For this review, take the finished solid that the model builds, in its own axes (mm). Face numbers are marked on the shaded views. A direction names the side the tool comes from. Coordinates: 2 decimals unless noted, no trailing zeros. Order: outer loops, then holes, each group sorted by start corner. A loop starts at its lowest first (then second) coordinate and runs counter-clockwise, first axis right, second up. Notation, with made-up numbers: (14, 2) -> (46, 2) arc R30 cw to (46, 36) -> close; hole circle Ø2 at (51, 79). An arc over 180 degrees is marked (long way). Answer as a JSON object with one key per item and string values. Group by question number.
1) Add section B-B, the plane z = 61. Write out the cut boundary in (x, y).
2) For pin 1 (5.5 mm diameter, centred on x = 36.5, y = 13.5, fed in from +Z); pin 2 (12 mm diameter, centred on y = -9, z = 47.5, fed in from -X); pin 3 (8 mm diameter, centred on y = -12.5, z = 17, fed in from -X); pin 4 (4 mm diameter, centred on x = 54, z = 52.5, fed in from -Y), all flat-tipped, find the tip position at first contact; note any pin that passes through.
3) Draft analysis for pull direction X (two halves, no side actions). For the marked faces 4, 5, 6 and 7, state which applies: +X half, -X half, draft (parallel to the pull), parting line (faces both ways), or undercut.
4) Wall thickness on L1, parallel to Y at x = 35, z = 22; L2, parallel to Y at x = 9, z = 38; L3, parallel to X at y = 9, z = 58: over which ranges is each line inside the solid? List them lowest first.
5) Add section D-D, the plane x = 32.5. Write out the cut boundary in (y, z).
6) Add section C-C, the plane y = -20.5. Write out the cut boundary in (x, z).
7) Machinability: for the marked faces 1, 2 and 3, which of the approach directions +Z, -Z, +X, -X, +Y, -Y give a long, thin tool a straight path to every point of the face, cutting with its end or side? Answer none if there is none.
8) Add section A-A, the plane z = 29. Write out the cut boundary in (x, y), then the cut area to 3 significant figures.
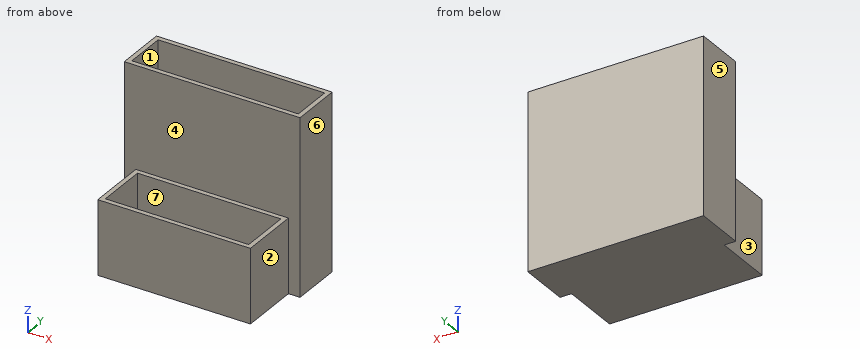
from build123d import *

# Parameters (mm, degrees)
SKETCH_W        = 76
SKETCH_H        = 22
PAD_DEPTH       = 76
SKETCH001_W     = 66
SKETCH001_H     = 26
PAD001_DEPTH    = 32
SKETCH002_W     = 62
SKETCH002_H     = 22
POCKET_DEPTH    = 30
SKETCH003_W     = 72
SKETCH003_H     = 18
POCKET001_DEPTH = 74


with BuildPart() as part:
    # Sketch → Pad (new body)
    with BuildSketch(Plane.XY):
        with Locations((38, 11)):
            Rectangle(SKETCH_W, SKETCH_H)
    extrude(amount=PAD_DEPTH)

    # Sketch001 → Pad001 (join)
    with BuildSketch(Plane.XY):
        with Locations((38, -13)):
            Rectangle(SKETCH001_W, SKETCH001_H)
    extrude(amount=PAD001_DEPTH)

    # Sketch002 (on Face4 of Pad001) → Pocket (cut)
    with BuildSketch(Plane.XY.offset(32)):
        with Locations((38, -13)):
            Rectangle(SKETCH002_W, SKETCH002_H)
    extrude(amount=-POCKET_DEPTH, mode=Mode.SUBTRACT)

    # Sketch003 (on Face7 of Pocket) → Pocket001 (cut)
    with BuildSketch(Plane.XY.offset(76)):
        with Locations((38, 11)):
            Rectangle(SKETCH003_W, SKETCH003_H)
    extrude(amount=-POCKET001_DEPTH, mode=Mode.SUBTRACT)


solid = part.part
Output values:
{
 "1": {"outline": "(0, 0) -> (76, 0) -> (76, 22) -> (0, 22) -> close; hole (2, 2) -> (74, 2) -> (74, 20) -> (2, 20) -> close"},
 "2": {"pin 1": "stops at z = 2", "pin 2": "passes through", "pin 3": "stops at x = 5", "pin 4": "stops at y = 0"},
 "3": {"face 4": "draft", "face 5": "-X half", "face 6": "+X half", "face 7": "undercut"},
 "4": {"L1": "y = -26 to -24, -2 to 2, 20 to 22", "L2": "y = 0 to 2, 20 to 22", "L3": "x = 0 to 2, 74 to 76"},
 "5": {"outline": "(-26, 0) -> (22, 0) -> (22, 76) -> (20, 76) -> (20, 2) -> (2, 2) -> (2, 76) -> (0, 76) -> (0, 32) -> (-2, 32) -> (-2, 2) -> (-24, 2) -> (-24, 32) -> (-26, 32) -> close"},
 "6": {"outline": "(5, 0) -> (71, 0) -> (71, 32) -> (69, 32) -> (69, 2) -> (7, 2) -> (7, 32) -> (5, 32) -> close"},
 "7": {"face 1": "+Z", "face 2": "+Z, -Z, +X, -Y", "face 3": "+Z, -Z, -X, -Y"},
 "8": {"outline": "(0, 0) -> (5, 0) -> (5, -26) -> (71, -26) -> (71, 0) -> (76, 0) -> (76, 22) -> (0, 22) -> close; hole (2, 2) -> (74, 2) -> (74, 20) -> (2, 20) -> close; hole (7, -24) -> (69, -24) -> (69, -2) -> (7, -2) -> close", "area": "728 mm²"}
}
